Geometry: final body of the model. Coordinates: model frame, mm. Coordinates: 2 decimals unless noted, no trailing zeros. Write each loop counter-clockwise with the first axis right and the second up, starting at its lowest first coordinate (ties: lowest second). Pieces come first, ordered by that corner, then holes.
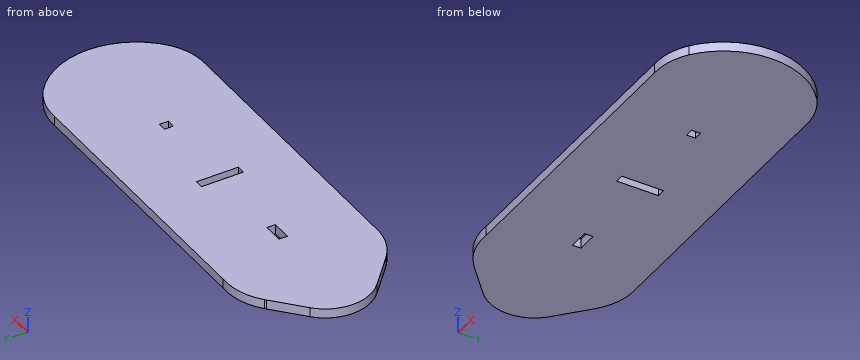
from build123d import *

# Parameters (mm, degrees)
F0_W     = 10
F0_H     = 4.2
F0_W_2   = 4.2
F0_H_2   = 20.833439
F0_H_3   = 4.413291
F1_DEPTH = 4.7


with BuildPart() as f1:
    # F0 (on Top) → F1 (new body)
    with BuildSketch(Plane.XY):
        with BuildLine():
            Line((77.899866, 37.688946), (-61.590597, 37.688946))
            ThreePointArc((-61.590597, 37.688946), (-73.325816, 36.25533), (-83.589011, 30.386986))
            Line((-83.589011, 30.386986), (-84.255223, 29.786773))
            Line((-84.255223, 29.786773), (-98.703748, 16.769597))
            ThreePointArc((-98.703748, 16.769597), (-106.083018, 0.188949), (-98.703748, -16.3917))
            Line((-98.703748, -16.3917), (-83.589011, -30.009089))
            ThreePointArc((-83.589011, -30.009089), (-73.325816, -35.877432), (-61.590597, -37.311049))
            Line((-61.590597, -37.311049), (77.991385, -37.311049))
            ThreePointArc((77.991385, -37.311049), (87.872, -36.035201), (96.792933, -31.59997))
            ThreePointArc((96.792933, -31.59997), (112.514041, 0.188949), (96.792933, 31.977867))
            ThreePointArc((96.792933, 31.977867), (87.872, 36.413099), (77.991385, 37.688946))
            Line((77.991385, 37.688946), (77.899866, 37.688946))
        make_face()
        with Locations((-43.705713, 0.082303)):
            Rectangle(F0_W, F0_H, mode=Mode.SUBTRACT)
        with Locations((3.496545, 0.188949)):
            Rectangle(F0_W_2, F0_H_2, mode=Mode.SUBTRACT)
        with Locations((47.798803, 0.188948)):
            Rectangle(F0_W_2, F0_H_3, mode=Mode.SUBTRACT)
        with BuildLine():
            Line((-84.255223, 29.786773), (-83.589011, 30.386986))
            ThreePointArc((-83.589011, 30.386986), (-83.924366, 30.089376), (-84.255223, 29.786773))
        make_face()
    extrude(amount=F1_DEPTH)


solid = f1.part
Item 1: Section C-C, the plane x = 89.5. Output: boundary loops of the cut face in (y, z), plus the area to 3 significant figures.
Derived:
outline: (-35.49, 0) - (35.87, 0) - (35.87, 4.7) - (-35.49, 4.7) - close
area: 335 mm2
Item 2: Material intervals for probe 1 along X at (y, z) = (-0.5, 4.15); probe 2 along Y at (x, z) = (-40.5, 0.35); probe 3 along Y at (x, z) = (49, 3.35), sorted ascending.
Derived:
probe 1: x = -106.07 to -48.71, -38.71 to 1.4, 5.6 to 45.7, 49.9 to 112.51
probe 2: y = -37.31 to -2.02, 2.18 to 37.69
probe 3: y = -37.31 to -2.02, 2.4 to 37.69
Item 3: Section D-D, the plane y = 26.5. Output: boundary loops of the cut face in (x, z), plus the area to 3 significant figures.
Derived:
outline: (-87.9, 0) - (102.64, 0) - (102.64, 4.7) - (-87.9, 4.7) - close
area: 896 mm2
Item 4: Pin query (flat end, axial travel): pin 1 (2 mm diameter, centred on x = 85, z = 2.5, fed in from +Y); pin 2 (2 mm diameter, centred on x = -4, z = 4, fed in from +Y); pin 3 (2 mm diameter, centred on x = 47.5, z = 1.5, fed in from -Y); pin 4 (1.3 mm diameter, centred on y = 0, z = 3, fed in from -X). Return the tip coordinate at first contact, or that it passes through.
Derived:
pin 1: stops at y = 37.31
pin 2: stops at y = 37.69
pin 3: stops at y = -37.31
pin 4: stops at x = -106.08
Item 5: Section B-B, the plane y = -5. Output: boundary loops of the cut face in (x, z), plus the area to 3 significant figures.
Derived:
outline: (-105.47, 0) - (1.4, 0) - (1.4, 4.7) - (-105.47, 4.7) - close; (5.6, 0) - (112.18, 0) - (112.18, 4.7) - (5.6, 4.7) - close
area: 1,000 mm2
Item 6: Section A-A, the plane z = 2.1. Output: boundary loops of the cut face in (x, y) (1 decimal), plus the area to 3 significant figures.
Derived:
outline: (-98.7, -16.4) - (-83.6, -30) arc R29.9 ccw to (-61.6, -37.3) - (78, -37.3) arc R30.1 ccw to (96.8, -31.6) arc R40 ccw to (96.8, 32) arc R30.1 ccw to (78, 37.7) - (-61.6, 37.7) arc R29.9 ccw to (-83.6, 30.4) arc R29.9 ccw to (-84.3, 29.8) - (-98.7, 16.8) arc R22.3 ccw to start; hole (-48.7, -2) - (-38.7, -2) - (-38.7, 2.2) - (-48.7, 2.2) - close; hole (1.4, -10.2) - (5.6, -10.2) - (5.6, 10.6) - (1.4, 10.6) - close; hole (45.7, -2) - (49.9, -2) - (49.9, 2.4) - (45.7, 2.4) - close
area: 14,800 mm2
